from build123d import *

# Parameters (mm, degrees)
BOSS_EXTRUDE1_DEPTH = 2
SKETCH2_W           = 2
SKETCH2_H           = 26
BOSS_EXTRUDE2_DEPTH = 24
BOSS_EXTRUDE3_DEPTH = 2
SKETCH4_R           = 4
CUT_EXTRUDE1_DEPTH  = 2
BOSS_EXTRUDE4_DEPTH = 26
CUT_EXTRUDE2_DEPTH  = 26
BOSS_EXTRUDE5_DEPTH = 2
SKETCH8_R           = 7.515013345
SKETCH8_R_2         = 4.48835621
BOSS_EXTRUDE6_DEPTH = 4
SKETCH9_R           = 3
CUT_EXTRUDE3_DEPTH  = 10
SKETCH10_R          = 4
CUT_EXTRUDE4_DEPTH  = 10
SKETCH11_R          = 4
SKETCH11_R_2        = 3
BOSS_EXTRUDE7_DEPTH = 7
SKETCH12_R          = 4
BOSS_EXTRUDE8_DEPTH = 1
SKETCH13_W          = 5
SKETCH13_H          = 10
CUT_EXTRUDE5_DEPTH  = 10
SKETCH14_W          = 5
SKETCH14_H          = 10
CUT_EXTRUDE6_DEPTH  = 4


with BuildPart() as part:
    # Sketch1 → Boss-Extrude1 (new body)
    with BuildSketch(Plane(origin=(0, 0, 0), x_dir=(1, 0, 0), z_dir=(0, 1, 0))):
        with BuildLine():
            Line((40, 13), (0, 13))
            ThreePointArc((0, 13), (-13, 0), (0, -13))
            Line((0, -13), (40, -13))
            Line((40, -13), (40, 13))
        make_face()
    extrude(amount=BOSS_EXTRUDE1_DEPTH)

    # Sketch2 → Boss-Extrude2 (add)
    with BuildSketch(Plane(origin=(0, 2, 0), x_dir=(1, 0, 0), z_dir=(0, 1, 0))):
        with Locations((39, 0)):
            Rectangle(SKETCH2_W, SKETCH2_H)
    extrude(amount=BOSS_EXTRUDE2_DEPTH)

    # Sketch3 → Boss-Extrude3 (add)
    with BuildSketch(Plane(origin=(0, 26, 0), x_dir=(1, 0, 0), z_dir=(0, 1, 0))):
        with BuildLine():
            Line((40, -13), (0, -13))
            ThreePointArc((0, -13), (-13, 0), (0, 13))
            Line((0, 13), (40, 13))
            Line((40, 13), (40, -13))
        make_face()
    extrude(amount=BOSS_EXTRUDE3_DEPTH)

    # Sketch4 → Cut-Extrude1 (cut)
    with BuildSketch(Plane(origin=(40, 0, 0), x_dir=(0, 0, -1), z_dir=(1, 0, 0))):
        with Locations((0, 14)):
            Circle(SKETCH4_R)
    extrude(amount=-CUT_EXTRUDE1_DEPTH, mode=Mode.SUBTRACT)

    # Sketch5 → Boss-Extrude4 (add)
    with BuildSketch(Plane.XY.offset(13)):
        Polygon((38, 5), (34, 2), (31.333333333, 0), (31.333333333, 2), (40, 8.5), (40, 6.5), align=None)
        Polygon((40, 21.5), (38, 23), (34, 26), (31.333333333, 28), (31.333333333, 26), (40, 19.5), align=None)
    extrude(amount=-BOSS_EXTRUDE4_DEPTH)

    # Sketch6 → Cut-Extrude2 (cut)
    with BuildSketch(Plane.XY.offset(13)):
        Polygon((38, 5), (31.333333333, 0), (40, 0), (40, 6.5), align=None)
        Polygon((40, 28), (40, 21.5), (38, 23), (31.333333333, 28), align=None)
    extrude(amount=-CUT_EXTRUDE2_DEPTH, mode=Mode.SUBTRACT)

    # Sketch7 → Boss-Extrude5 (add)
    with BuildSketch(Plane.XY.offset(13)):
        Polygon((40, 21.5), (31.333333333, 28), (20.333333333, 28), (20.333333333, 0), (31.333333333, 0), (40, 6.5), align=None)
    boss_extrude5 = extrude(amount=BOSS_EXTRUDE5_DEPTH)

    # Mirror1: Boss-Extrude5 across plane
    add(boss_extrude5.mirror(Plane.XY))

    # Sketch8 → Boss-Extrude6 (add)
    with BuildSketch(Plane.ZY.offset(-38)):
        with Locations(Location((0, 14, 0), (0, 0, 111.335065793))):
            Circle(SKETCH8_R)
        with Locations((0, 14)):
            Circle(SKETCH8_R_2, mode=Mode.SUBTRACT)
    extrude(amount=BOSS_EXTRUDE6_DEPTH)

    # Sketch9 → Cut-Extrude3 (cut)
    with BuildSketch(Plane.XZ):
        with Locations(Location((0, 0, 0), (0, 0, 270))):
            Circle(SKETCH9_R)
    extrude(amount=-CUT_EXTRUDE3_DEPTH, mode=Mode.SUBTRACT)

    # Sketch10 → Cut-Extrude4 (cut)
    with BuildSketch(Plane(origin=(0, 28, 0), x_dir=(1, 0, 0), z_dir=(0, 1, 0))):
        with Locations(Location((0, 0, 0), (0, 0, 270))):
            Circle(SKETCH10_R)
    extrude(amount=-CUT_EXTRUDE4_DEPTH, mode=Mode.SUBTRACT)

    # Sketch11 → Boss-Extrude7 (add)
    with BuildSketch(Plane.XZ):
        with Locations(Location((0, 0, 0), (0, 0, 90))):
            Circle(SKETCH11_R)
        with Locations(Location((0, 0, 0), (0, 0, 270))):
            Circle(SKETCH11_R_2, mode=Mode.SUBTRACT)
    extrude(amount=BOSS_EXTRUDE7_DEPTH)

    # Sketch12 → Boss-Extrude8 (add)
    with BuildSketch(Plane.XZ.offset(7)):
        with Locations(Location((0, 0, 0), (0, 0, 90))):
            Circle(SKETCH12_R)
    extrude(amount=BOSS_EXTRUDE8_DEPTH)

    # Sketch13 → Cut-Extrude5 (cut)
    with BuildSketch(Plane.XY.offset(15)):
        with Locations((27.833333333, 14)):
            Rectangle(SKETCH13_W, SKETCH13_H)
    extrude(amount=-CUT_EXTRUDE5_DEPTH, mode=Mode.SUBTRACT)

    # Sketch14 → Cut-Extrude6 (cut)
    with BuildSketch(Plane(origin=(0, 0, -15), x_dir=(-1, 0, 0), z_dir=(0, 0, -1))):
        with Locations((-27.833333333, 14)):
            Rectangle(SKETCH14_W, SKETCH14_H)
    extrude(amount=-CUT_EXTRUDE6_DEPTH, mode=Mode.SUBTRACT)


solid = part.part
Here's how the part is built. I have some questions about the finished solid (model axes, mm). A direction names the side the tool comes from. Round coordinates to 2 decimals unless told otherwise and drop trailing zeros. Loops run counter-clockwise (first coordinate to the right, second up) from the corner with the lowest first, then second, coordinate; pieces in that order, holes last. Notation, with made-up numbers: M 65.5,17 L 94.5,17 A26 ccw 94.5,32 Z; hole C 57.25,47 d9. An arc over 180 degrees is marked long. Write each question's results on one line, items separated by ' | '. Start each with the question number.
(1) If I drill on probe 1 along Y at (x, z) = (-1, 12.5); probe 2 along Y at (x, z) = (34.8, 0); probe 3 along Z at (x, y) = (32.5, 21), over which ranges is the centre line in solid material (lowest first)? Write a range as from..to.
(2) Thinking about a two-plate mould opening in Z: for faces 6 (the flat face through (38, 14, -9)), 7 (the flat face through (28, 19, 14)), 8 (the cylindrical face through (-13, 27, 0)), which applies, pulls with the +Z half, pulls with the -Z half, needs draft (parallel to the pull), parting line crosses it, or undercut?
(3) I want a section at D-D (z = 10). Please give me the cut outline in (x, y), then the cut area to 3 significant figures.
(4) I want a section at B-B (y = 14). Please give me the cut outline in (x, z), then the cut area to 3 significant figures.
(5) Will these pins go through, and if not, where does the flat tip stop? P1, Ø1, axis at y = 14.5, z = 14, coming from the -X side; P2, Ø7, axis at y = 14, z = 0, coming from the +X side; P3, Ø2, axis at x = -1, y = -3.5, coming from the +Z side; P4, Ø10, axis at y = 13, z = 1, coming from the -X side.
(6) I want a section at A-A (x = 36). Please give me the cut outline in (y, z).
(7) I want a section at C-C (x = 5). Please give me the cut outline in (y, z).
(8) On a 3-axis mill with a long thin cutter (end or side, diameter ignored), from which of +Z, -Z, +X, -X, +Y, -Y can I reach the whole of each face in a straight line? I mean faces 1 (the flat face through (10, 1, -13)), 2 (the flat face through (38, 17, 3)), 3 (the flat face through (28, 9, 14)), 4 (the cylindrical face through (3.905, -3.944, -0.867)), 5 (the flat face through (0, -7, 0)). Say none if no direction works.
Solved:
1) probe 1: y = 0..2, 26..28 | probe 2: y = 2.6..4.6, 6.48..9.51, 18.49..21.52, 23.4..25.4 | probe 3: z = -15..-13, 13..15
2) face 6: undercut | face 7: needs draft | face 8: parting line crosses it
3) outline: M -8.31,0 L 31.33,0 L 40,6.5 L 40,21.5 L 31.33,28 L -8.31,28 L -8.31,26 L 31.33,26 L 38,21 L 38,7 L 31.33,2 L -8.31,2 Z | area: 218 mm²
4) outline: M 20.33,-15 L 25.33,-15 L 25.33,-13 L 20.33,-13 Z; M 20.33,13 L 25.33,13 L 25.33,15 L 20.33,15 Z; M 30.33,-15 L 40,-15 L 40,-4 L 38,-4 L 38,-4.49 L 34,-4.49 L 34,-7.52 L 38,-7.52 L 38,-13 L 30.33,-13 Z; M 30.33,13 L 38,13 L 38,7.52 L 34,7.52 L 34,4.49 L 38,4.49 L 38,4 L 40,4 L 40,15 L 30.33,15 Z | area: 119 mm²
5) P1: stops at x = 20.33 | P2: passes through | P3: stops at z = 4 | P4: stops at x = 34
6) outline: M 3.5,-15 L 24.5,-15 L 24.5,15 L 3.5,15 Z; C 14,0 d15.03; hole M 5.5,-13 L 22.5,-13 L 22.5,13 L 5.5,13 Z; hole C 14,0 d8.98
7) outline: M 0,-13 L 2,-13 L 2,13 L 0,13 Z; M 26,-13 L 28,-13 L 28,13 L 26,13 Z
8) face 1: -Z, -X, +Y, -Y | face 2: -X | face 3: +Z, -Z | face 4: -Y | face 5: +Y
